Could you check a few things on this drawing? It's one solid part, dimensions in mm from its lowest x, y, z. Give positions to 0.01 mm unless a question says otherwise; leave off trailing zeros. Loops run counter-clockwise (first coordinate to the right, second up) from the corner with the lowest first, then second, coordinate; pieces in that order, holes last. Notation, with made-up numbers: (41, 40.5) -> (73, 40.5) arc R13 cw to (73, 64.5) -> close; hole circle Ø10 at (74, 51). An arc over 180 degrees is marked (long way). Use CSV: the item, a comma, the result in double quotes.
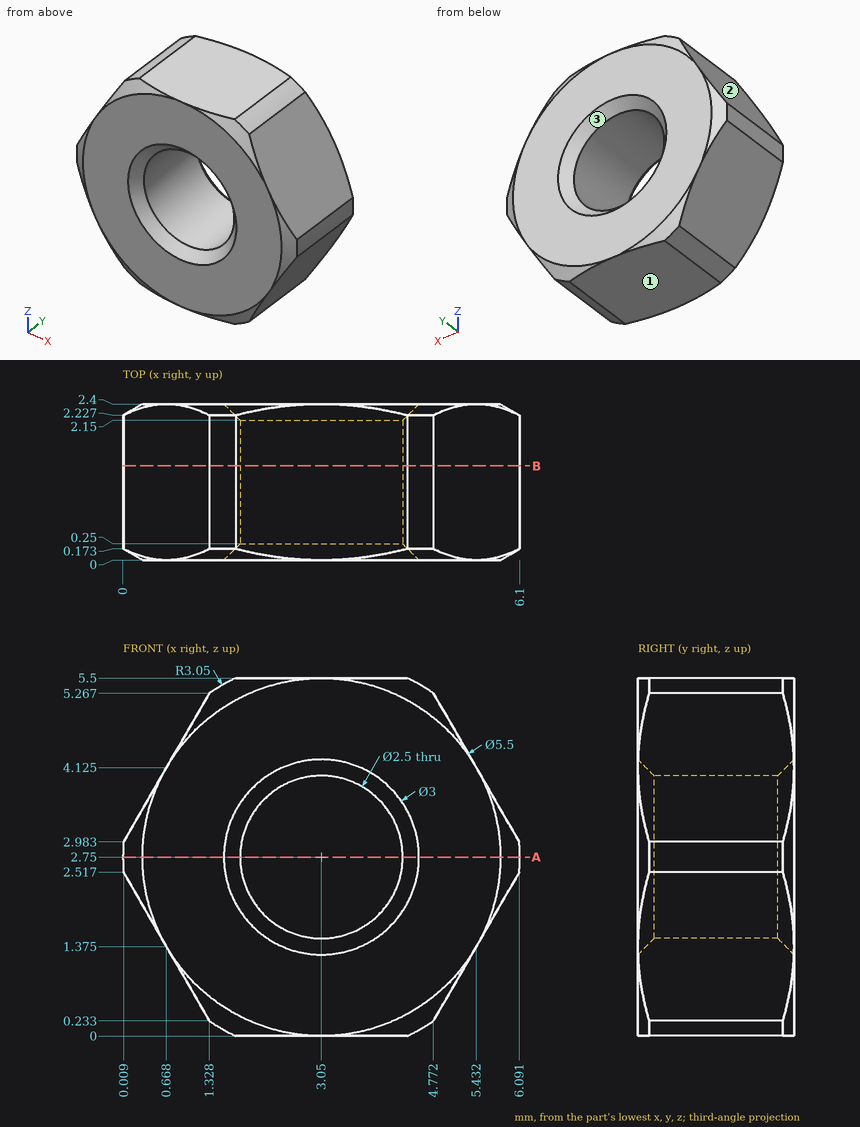
(1) If we section it at A-A, the plane z = 2.75: Write out the boundary of the cut face in (x, y).
Answer sheet:
outline,"(0, 0.17) -> (0.3, 0) -> (1.55, 0) -> (1.8, 0.25) -> (1.8, 2.15) -> (1.55, 2.4) -> (0.3, 2.4) -> (0, 2.23) -> close; (4.3, 0.25) -> (4.55, 0) -> (5.8, 0) -> (6.1, 0.17) -> (6.1, 2.23) -> (5.8, 2.4) -> (4.55, 2.4) -> (4.3, 2.15) -> close"
(2) We'd pull the mould along X, two halves only. Please class the marked faces 1, 2 and 3: released by +X, released by -X, zero draft, split by the parting line, or undercut.
Answer sheet:
face 1,"zero draft"
face 2,"released by -X"
face 3,"undercut"
(3) If I drill on L1, parallel to Z at x = 3.05, y = 0.6; L2, parallel to Z at x = 2.5, y = 1.85; L3, parallel to Z at x = 5.5, y = 0.4 (1 decimal), over which ranges is the centre line in solid material (lowest first)? Write a range as from..to.
Answer sheet:
L1,"z = 0..1.5, 4..5.5"
L2,"z = 0..1.63, 3.87..5.5"
L3,"z = 1.5..4"
(4) If we section it at B-B, the plane y = 1.45: Write out the boundary of the cut face in (x, z).
Answer sheet:
outline,"(0.01, 2.52) -> (1.33, 0.23) arc R3.05 ccw to (1.73, 0) -> (4.37, 0) arc R3.05 ccw to (4.77, 0.23) -> (6.09, 2.52) arc R3.05 ccw to (6.09, 2.98) -> (4.77, 5.27) arc R3.05 ccw to (4.37, 5.5) -> (1.73, 5.5) arc R3.05 ccw to (1.33, 5.27) -> (0.01, 2.98) arc R3.05 ccw to start; hole circle Ø2.5 at (3.05, 2.75)"
